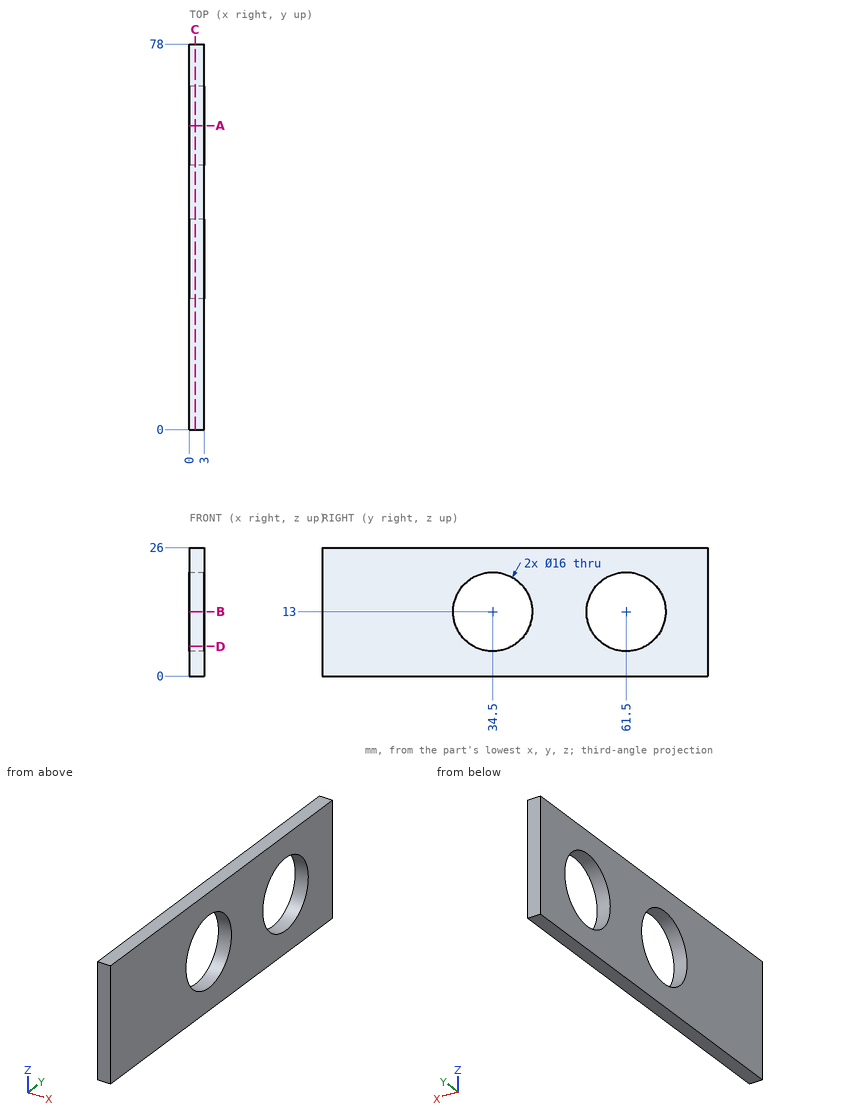
Drawing for the job (mm, zero at the part's lowest x, y, z). Round coordinates to 2 decimals unless told otherwise and drop trailing zeros. Order: outer loops, then holes, each group sorted by start corner. A loop starts at its lowest first (then second) coordinate and runs counter-clockwise, first axis right, second up.
Item 1: Saw through at C-C on x = 1.15. Write the cut outline in (y, z), then the cut area to 3 significant figures.
Item 2: Pin check, flat tips, straight feed: pin 1 (12 mm diameter, centred on y = 56, z = 15.5, fed in from +X); pin 2 (9.5 mm diameter, centred on y = 61.5, z = 13, fed in from -X). Stop position of each tip, or through.
Item 3: Saw through at D-D on z = 6. Write the cut outline in (x, y), then the cut area to 3 significant figures.
Item 4: Probe line 1 along Y through (x, z) = (1.2, 12.5); line 2 along Y through (x, z) = (0.2, 10); line 3 along Z through (x, y) = (2.15, 67). List the from-to ranges inside material, lowest first.
Item 5: Saw through at A-A on y = 61.5. Write the cut outline in (x, z), then the cut area to 3 significant figures.
Item 6: Saw through at B-B on z = 13. Write the cut outline in (x, y).
Reported:
1. outline: (0, 0) - (78, 0) - (78, 26) - (0, 26) - close; hole circle Ø16 at (34.5, 13); hole circle Ø16 at (61.5, 13)
1. area: 1,630 mm2
2. pin 1: stops at x = 3
2. pin 2: passes through
3. outline: (0, 0) - (3, 0) - (3, 30.63) - (0, 30.63) - close; (0, 38.37) - (3, 38.37) - (3, 57.63) - (0, 57.63) - close; (0, 65.37) - (3, 65.37) - (3, 78) - (0, 78) - close
3. area: 188 mm2
4. line 1: y = 0 to 26.52, 42.48 to 53.52, 69.48 to 78
4. line 2: y = 0 to 27.08, 41.92 to 54.08, 68.92 to 78
4. line 3: z = 0 to 7.19, 18.81 to 26
5. outline: (0, 0) - (3, 0) - (3, 5) - (0, 5) - close; (0, 21) - (3, 21) - (3, 26) - (0, 26) - close
5. area: 30.0 mm2
6. outline: (0, 0) - (3, 0) - (3, 26.5) - (0, 26.5) - close; (0, 42.5) - (3, 42.5) - (3, 53.5) - (0, 53.5) - close; (0, 69.5) - (3, 69.5) - (3, 78) - (0, 78) - close
